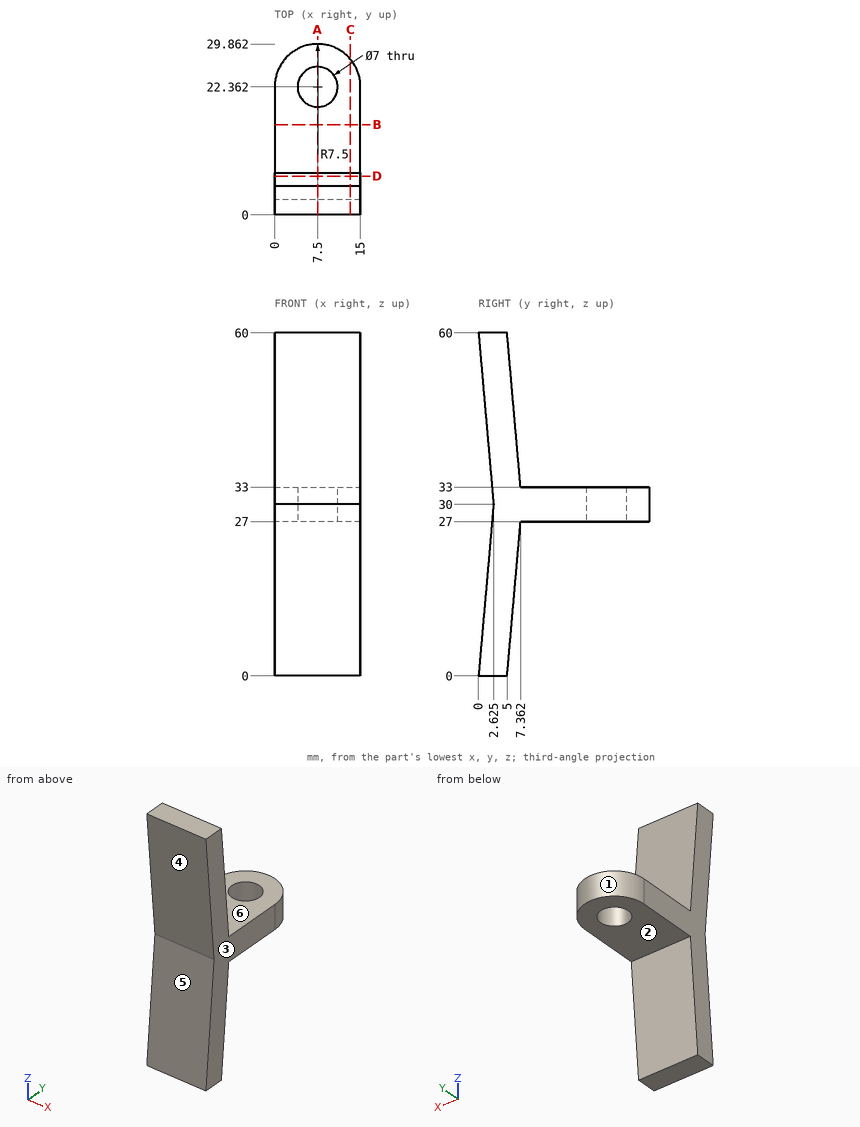
The figure shows three views and two pictorial views of one solid part (mm, origin at its lowest corner). Answer the questions. A direction names the side the tool comes from. Coordinates: 2 decimals unless noted, no trailing zeros. Loops run counter-clockwise (first coordinate to the right, second up) from the corner with the lowest first, then second, coordinate; pieces in that order, holes last. Notation, with made-up numbers: (-29.5, 9.25) -> (22.5, 9.25) arc R32 cw to (22.5, 41.25) -> close; hole circle Ø3 at (53, 40.5). An arc over 180 degrees is marked (long way). Use one line per item in the form item = value. Start each with the question number.
Item 1: The part is cut by section B-B on y = 15.75. Determine the outline of the cut face in (x, z).
Item 2: A tool of negligible diameter and unlimited length cuts with its end or side. For the marked faces 1 and 2, from which of +Z, -Z, +X, -X, +Y, -Y can it reach the whole face along a straight path? Write none if from no direction.
Item 3: Consider L1, parallel to Z at x = 3.5, y = 11; L2, parallel to Y at x = 7.5, z = 31.05; L3, parallel to Y at x = 14.25, z = 36.5. Determine where each line is inside the solid, lowest interval first. Write a range as [from, to].
Item 4: The part is cut by section C-C on x = 13.25. Determine the outline of the cut face in (y, z) (1 decimal), then the cut area to 3 significant figures.
Item 5: Flat-ended cylindrical pins translate along their axes: pin 1 Ø7.5 at (x, y) = (4.5, 13.5) entering from -Z; pin 2 Ø4 at (x, z) = (12.5, 34.5) entering from -Y; pin 3 Ø1 at (x, y) = (7.5, 21) entering from +Z; pin 4 Ø8 at (x, y) = (7.5, 22.36) entering from +Z. Find the tip coordinate at first contact, or state that the pin passes through.
Item 6: The mould has two halves that part along Z. Classify the marked faces 3, 4, 5 and 6: released by +Z, released by -Z, zero draft, split by the parting line, or undercut.
Item 7: The part is cut by section A-A on x = 7.5. Determine the outline of the cut face in (y, z) (1 decimal), then the cut area to 3 significant figures.
Item 8: The part is cut by section D-D on y = 6.75. Determine the outline of the cut face in (x, z), then the cut area to 3 significant figures.
Answer key:
q1.outline = (0, 27) -> (15, 27) -> (15, 33) -> (0, 33) -> close
q2.face_1 = +Z, -Z, +Y
q2.face_2 = -Z, +X, -X, +Y
q3.L1 = [27, 33]
q3.L2 = [2.53, 18.86], [25.86, 29.86]
q3.L3 = [2.06, 7.06]
q4.outline = (0, 0) -> (5, 0) -> (7.4, 27) -> (27.2, 27) -> (27.2, 33) -> (7.4, 33) -> (5, 60) -> (0, 60) -> (2.6, 30) -> close
q4.area = 418 mm2
q5.pin_1 = 27
q5.pin_2 = 2.06
q5.pin_3 = through
q5.pin_4 = 33
q6.face_3 = zero draft
q6.face_4 = undercut
q6.face_5 = undercut
q6.face_6 = released by +Z
q7.outline = (0, 0) -> (5, 0) -> (7.4, 27) -> (18.9, 27) -> (18.9, 33) -> (7.4, 33) -> (5, 60) -> (0, 60) -> (2.6, 30) -> close; (25.9, 27) -> (29.9, 27) -> (29.9, 33) -> (25.9, 33) -> close
q7.area = 392 mm2
q8.outline = (0, 20) -> (15, 20) -> (15, 40) -> (0, 40) -> close
q8.area = 300 mm2
